The listing builds one solid part. Answer for the finished solid, in the listing's coordinates (mm). A direction names the side the tool comes from. Give positions to 0.01 mm unless a question says otherwise; leave off trailing zeros. Order: outer loops, then holes, each group sorted by start corner. A loop starts at its lowest first (then second) coordinate and runs counter-clockwise, first axis right, second up. Notation, with made-up numbers: (23.5, 25.25) - (37.5, 25.25) arc R26 cw to (37.5, 60.25) - close; hole circle Ø10 at (49.25, -39). An arc over 180 degrees is marked (long way). Answer as a JSON object with one key per item and string values. Group by question number.
Q1. A cutting plane is placed at C-C, the plane x = 62.5. Give the vertices of the cut face in (y, z).
Q2. Given pin 1 (1.5 mm diameter, centred on x = 119.5, z = -13.5, fed in from -Y); pin 2 (13.5 mm diameter, centred on y = 0, z = 0, fed in from +X); pin 3 (1.5 mm diameter, centred on x = 101, z = 6.5, fed in from -Y); pin 4 (1.5 mm diameter, centred on x = 77, y = -5, fed in from +Z), each flat-ended and moving along its own axis, determine where each tip first touches the part or whether it passes through.
Q3. Consider line 1 (Y direction, x = 176, z = 0); line 2 (Y direction, x = 95, z = 0). Determine where each line is inside the solid, lowest interval first.
Q4. For faces 4 (the face through (163.27, -2.38, -10.74)), 5 (the face through (70.98, 12.932, -5.362)), 6 (the face through (0, -12, 8)), determine the directions among +Z, -Z, +X, -X, +Y, -Y from which every point of the face is accessible in a straight line to the end or side of a thin tool.
Q5. The mould has two halves that part along Z. Classify faces 1 (the face through (70.98, 16.72, 5.26)), 2 (the face through (184, -2, -7.4)), 3 (the face through (164.28, 7.13, 2.24)): released by +Z, released by -Z, zero draft, split by the parting line, or undercut.
Q6. A cutting plane is placed at A-A, the plane z = 0. Give the vertices of the cut face in (x, y), and give its area (3 significant figures).
Autodesk Inventor part; units mm, degrees
ref_plane "YZ Plane" through (0, 0, 0) normal (1, 0, 0) x (0, 1, 0)
ref_plane "XZ Plane" through (0, 0, 0) normal (0, 1, 0) x (-1, 0, 0)
ref_plane "XY Plane" through (0, 0, 0) normal (0, 0, 1) x (1, 0, 0)
sketch "Boceto1" plane through (0, 0, 0) normal (0, 0, 1) x (1, 0, 0)
  line L0 (0, 0) -> (0, 17.526)
  line L1 (0, 17.526) -> (140, 17.526)
  line L2 (140, 17.526) -> (144, 11)
  line L3 (144, 11) -> (184, 11)
  line L4 (184, 11) -> (184, 0)
  line L5 (144, 7.474) -> (184, 7.474)
  line L6 (184, 0) -> (0, 0)
  line L7 (0, 17.526) -> (0, 14)
  line L8 (0, 14) -> (140, 14)
  line L9 (144, 7.474) -> (140, 14)
  point P0 (0, 11.6562)
  dimension "d5" = 140
  dimension "d9" = 40
  dimension "d13" = 17.526
  dimension "d14" = 14
revolve "Revolución2" add sketch "Boceto1" angle 360 about axis through (184, 0, 0) along (-1, 0, 0) contours L0 L1 L2 L3 L4 L5 L9 L8
fillet "Empalme2" radius 2 1 edges at (184, -11, 0)
equation "\"d13\" = 0.5 * DintTub"
equation "\"d14\" = 0.5 * DIntTubTen"
properties material "Acero"
Reply:
{
 "1": {"outline": "circle Ø35.05 at (0, 0); hole circle Ø28 at (0, 0)"},
 "2": {"pin 1": "stops at y = -12.02", "pin 2": "passes through", "pin 3": "stops at y = -16.56", "pin 4": "stops at z = 17"},
 "3": {"line 1": "y = -11 to -7.47, 7.47 to 11", "line 2": "y = -17.53 to -14, 14 to 17.53"},
 "4": {"face 4": "+X", "face 5": "-X", "face 6": "+Z, -Z, -X, +Y, -Y"},
 "5": {"face 1": "split by the parting line", "face 2": "zero draft", "face 3": "undercut"},
 "6": {"outline": "(0, -17.53) - (140, -17.53) - (144, -11) - (182, -11) arc R2 ccw to (184, -9) - (184, -7.47) - (144, -7.47) - (140, -14) - (0, -14) - close; (0, 14) - (140, 14) - (144, 7.47) - (184, 7.47) - (184, 9) arc R2 ccw to (182, 11) - (144, 11) - (140, 17.53) - (0, 17.53) - close", "area": "1,300 mm^2"}
}
